from build123d import *

# Parameters (mm, degrees)
SKETCH1_W                 = 39
SKETCH1_H                 = 39
BOSS_EXTRUDE1_DEPTH       = 0.8
FILLET1_R                 = 0.5
SKETCH2_R                 = 1.1
CUT_EXTRUDE1_DEPTH        = 1.6
SKETCH3_W                 = 7
SKETCH3_H                 = 7
BOSS_EXTRUDE2_DEPTH       = 2
SKETCH4_W                 = 14
SKETCH4_H                 = 14
BOSS_EXTRUDE3_DEPTH       = 4
SKETCH5_W                 = 15
SKETCH5_H                 = 15
BOSS_EXTRUDE4_DEPTH       = 0.1
SKETCH6_R                 = 7.5
BOSS_EXTRUDE5_DEPTH       = 15
M12_CLEARANCE_HOLE1_D     = 13
M12_CLEARANCE_HOLE1_DEPTH = 15.1


with BuildPart() as part:
    # Sketch1 → Boss-Extrude1 (new, symmetric)
    with BuildSketch(Plane(origin=(0, 0, 0), x_dir=(1, 0, 0), z_dir=(0, 1, 0))):
        Rectangle(SKETCH1_W, SKETCH1_H)
    extrude(amount=BOSS_EXTRUDE1_DEPTH, both=True)

    # Fillet1
    fillet1_edges = [part.edges().sort_by_distance(p)[0] for p in [
        (19.5, 0, 19.5),
        (-19.5, 0, 19.5),
        (-19.5, 0, -19.5),
        (19.5, 0, -19.5),
    ]]
    fillet(fillet1_edges, radius=FILLET1_R)

    # Sketch2 → Cut-Extrude1 (cut)
    with BuildSketch(Plane(origin=(0, 0.8, 0), x_dir=(1, 0, 0), z_dir=(0, 1, 0))):
        with Locations(Location((-17.3, 17.3, 0), (0, 0, 270))):
            Circle(SKETCH2_R)
        with Locations(Location((-17.3, -17.3, 0), (0, 0, 90))):
            Circle(SKETCH2_R)
        with Locations(Location((17.3, -17.3, 0), (0, 0, 270))):
            Circle(SKETCH2_R)
        with Locations(Location((17.3, 17.3, 0), (0, 0, 90))):
            Circle(SKETCH2_R)
    extrude(amount=-CUT_EXTRUDE1_DEPTH, mode=Mode.SUBTRACT)

    # Sketch3 → Boss-Extrude2 (add)
    with BuildSketch(Plane(origin=(0, 0.8, 0), x_dir=(1, 0, 0), z_dir=(0, 1, 0))):
        Rectangle(SKETCH3_W, SKETCH3_H)
    extrude(amount=BOSS_EXTRUDE2_DEPTH)

    # Sketch4 → Boss-Extrude3 (add)
    with BuildSketch(Plane(origin=(0, 0.8, 0), x_dir=(1, 0, 0), z_dir=(0, 1, 0))):
        with BuildLine():
            Line((-2, 9.5), (-2, 7.5))
            Line((-2, 7.5), (-7.5, 7.5))
            Line((-7.5, 7.5), (-7.5, -7.5))
            Line((-7.5, -7.5), (-2, -7.5))
            Line((-2, -7.5), (-2, -9.5))
            ThreePointArc((-2, -9.5), (0, -11.5), (2, -9.5))
            Line((2, -9.5), (2, -7.5))
            Line((2, -7.5), (7.5, -7.5))
            Line((7.5, -7.5), (7.5, 7.5))
            Line((7.5, 7.5), (2, 7.5))
            Line((2, 7.5), (2, 9.5))
            ThreePointArc((2, 9.5), (0, 11.5), (-2, 9.5))
        make_face()
        Rectangle(SKETCH4_W, SKETCH4_H, mode=Mode.SUBTRACT)
    extrude(amount=BOSS_EXTRUDE3_DEPTH)

    # Sketch5 → Boss-Extrude4 (add)
    with BuildSketch(Plane(origin=(0, 4.8, 0), x_dir=(1, 0, 0), z_dir=(0, 1, 0))):
        Rectangle(SKETCH5_W, SKETCH5_H)
    extrude(amount=-BOSS_EXTRUDE4_DEPTH)

    # Sketch6 → Boss-Extrude5 (add)
    with BuildSketch(Plane(origin=(0, 4.8, 0), x_dir=(1, 0, 0), z_dir=(0, 1, 0))):
        with Locations(Location((0, 0, 0), (0, 0, 180))):
            Circle(SKETCH6_R)
    extrude(amount=BOSS_EXTRUDE5_DEPTH)

    # M12 Clearance Hole1
    with Locations(Plane(origin=(0, 19.8, 0), x_dir=(1, 0, 0), z_dir=(0, 1, 0))):
        with Locations((0, 0)):
            Hole(M12_CLEARANCE_HOLE1_D / 2, depth=M12_CLEARANCE_HOLE1_DEPTH)


solid = part.part
For this review, take the finished solid that the model builds, in its own axes (mm). A direction names the side the tool comes from. Give positions to 0.01 mm unless a question says otherwise; leave off trailing zeros. Order: outer loops, then holes, each group sorted by start corner. A loop starts at its lowest first (then second) coordinate and runs counter-clockwise, first axis right, second up. Notation, with made-up numbers: (75.5, 66) -> (83.5, 66) arc R15 cw to (83.5, 85) -> close; hole circle Ø11 at (-24, 49). An arc over 180 degrees is marked (long way). Write item = value, one per line.
1) Insertion check: pin 1 (1.6 mm diameter, centred on y = 2, z = -1, fed in from -X); pin 2 (0.6 mm diameter, centred on y = 3, z = 9, fed in from +X); pin 3 (8 mm diameter, centred on y = 9.5, z = 6, fed in from +X). Each pin has a flat end and moves straight along its axis. Give the tip position at first contact, or say it passes through.
Findings:
pin_1 = -7.5
pin_2 = 2
pin_3 = 7.23
2) Draft analysis for pull direction Z (two halves, no side actions). For faces 6 (the face through (5, 3, -7.5)), 7 (the face through (-16.879, 0.011, 16.284)), 8 (the face through (-2, 3, 8)), 9 (the face through (-16.97, 0.01, -16.25)), state which applies: pulls with the +Z half, pulls with the -Z half, needs draft (parallel to the pull), parting line crosses it, or undercut.
Findings:
face_6 = pulls with the -Z half
face_7 = undercut
face_8 = needs draft
face_9 = undercut
3) To check wall thickness, follow L1, parallel to X at y = 0.25, z = 17.3; L2, parallel to Y at x = 1, z = 6.5; L3, parallel to X at y = 2.75, z = 4.5. State the ranges of each line that lie inside material, in increasing order. Write a range as from..to.
Findings:
L1 = -19.5..-18.4, -16.2..16.2, 18.4..19.5
L2 = -0.8..0.8, 4.7..19.8
L3 = -7.5..-7, 7..7.5
4) We need section B-B, the plane x = 17.3. Give the boundary of the cut face in (y, z), and give its area (3 significant figures).
Findings:
outline = (-0.8, -19.5) -> (0.8, -19.5) -> (0.8, -18.4) -> (-0.8, -18.4) -> close; (-0.8, -16.2) -> (0.8, -16.2) -> (0.8, 16.2) -> (-0.8, 16.2) -> close; (-0.8, 18.4) -> (0.8, 18.4) -> (0.8, 19.5) -> (-0.8, 19.5) -> close
area = 55.4 mm^2
5) We need section C-C, the plane y = 17.75. Give the boundary of the cut face in (x, z), and give its area (3 significant figures).
Findings:
outline = circle Ø15 at (0, 0); hole circle Ø13 at (0, 0)
area = 44.0 mm^2
6) We need section D-D, the plane x = 0. Give the boundary of the cut face in (y, z).
Findings:
outline = (-0.8, -19.5) -> (0.8, -19.5) -> (0.8, -11.5) -> (4.8, -11.5) -> (4.8, -7.5) -> (19.8, -7.5) -> (19.8, -6.5) -> (4.7, -6.5) -> (4.7, -7) -> (0.8, -7) -> (0.8, -3.5) -> (2.8, -3.5) -> (2.8, 3.5) -> (0.8, 3.5) -> (0.8, 7) -> (4.7, 7) -> (4.7, 6.5) -> (19.8, 6.5) -> (19.8, 7.5) -> (4.8, 7.5) -> (4.8, 11.5) -> (0.8, 11.5) -> (0.8, 19.5) -> (-0.8, 19.5) -> close
7) For faces 1 (the face through (3.5, 2, 0)), 2 (the face through (-2, 3, -9)), 3 (the face through (0, 0.8, -5)), 4 (the face through (0, 4.8, -8)), 5 (the face through (2, 3, 9)), list the 3-axis set-ups (+Z, -Z, +X, -X, +Y, -Y) from which the entire face can be reached by the end or side of a thin tool; tool diameter is ignored.
Findings:
face_1 = +Y
face_2 = -Z, -X, +Y
face_3 = none
face_4 = -Z, +Y
face_5 = +Z, +X, +Y
8) We need section A-A, the plane z = 17.3. Give the boundary of the cut face in (x, y).
Findings:
outline = (-19.5, -0.8) -> (-18.4, -0.8) -> (-18.4, 0.8) -> (-19.5, 0.8) -> close; (-16.2, -0.8) -> (16.2, -0.8) -> (16.2, 0.8) -> (-16.2, 0.8) -> close; (18.4, -0.8) -> (19.5, -0.8) -> (19.5, 0.8) -> (18.4, 0.8) -> close
